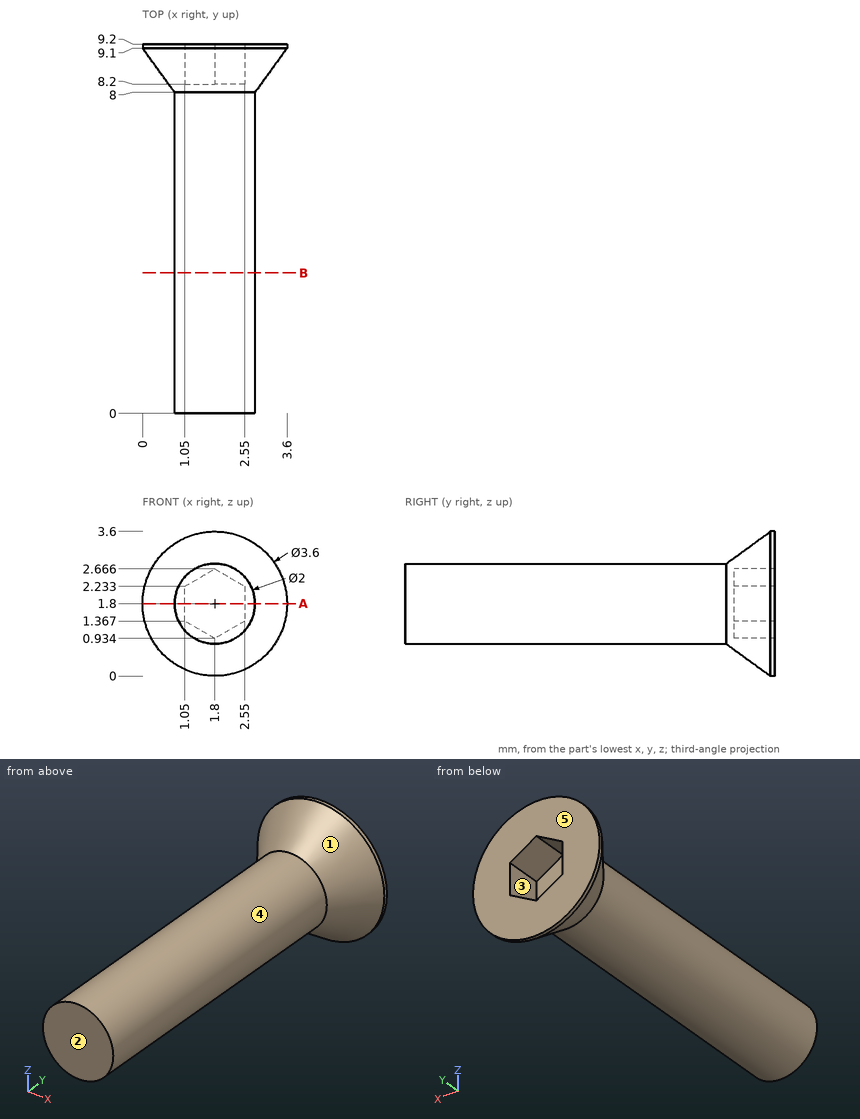
Here's the drawing with two shaded views (mm, measured from the low corner). I have some questions. A direction names the side the tool comes from. Give positions to 0.01 mm unless a question says otherwise; leave off trailing zeros. Loops run counter-clockwise (first coordinate to the right, second up) from the corner with the lowest first, then second, coordinate; pieces in that order, holes last. Notation, with made-up numbers: (0, 57) - (28, 57) arc R14 ccw to (28, 80) - close; hole circle Ø2 at (-27, 47). An arc over 180 degrees is marked (long way). Answer in a Markdown table with one row per item. Add a question column.
Q1. We'd pull the mould along Z, two halves only. Please class the marked faces 1, 2 and 3: +Z half, -Z half, draft (parallel to the pull), parting line (faces both ways), or undercut.
Q2. If we section it at B-B (y = 3.5): List the corners of the cut face in (x, z) for me.
Q3. If we section it at A-A (z = 1.8): List the corners of the cut face in (x, y) for me, plus the area to 3 significant figures.
Q4. Please list where these lines run through material, in increasing order: L1, parallel to Y at x = 1.8, z = 1.85; L2, parallel to X at y = 6, z = 2.3; L3, parallel to Y at x = 2.6, z = 2.6. Write a range as from..to.
Q5. For pin 1 (1 mm diameter, centred on y = 4.5, z = 0.5, fed in from -X); pin 2 (1.5 mm diameter, centred on x = 1, y = 4.5, fed in from +Z); pin 3 (0.5 mm diameter, centred on x = 2, z = 2, fed in from +Y), each with a flat end and sliding along its axis, tell me the tip position at first contact or that it passes through.
Q6. Which directions (+Z, -Z, +X, -X, +Y, -Y) give clear straight access to the entire face, cutting with the end or side of a thin tool? Please do the marked faces 4 and 5.
The answers:
| question | item | result |
|---|---|---|
| 1 | face 1 | parting line |
| 1 | face 2 | draft |
| 1 | face 3 | undercut |
| 2 | outline | circle Ø2 at (1.8, 1.8) |
| 3 | outline | (0, 9.1) - (0.8, 8) - (0.8, 0) - (2.8, 0) - (2.8, 8) - (3.6, 9.1) - (3.6, 9.2) - (2.55, 9.2) - (2.55, 8.2) - (1.05, 8.2) - (1.05, 9.2) - (0, 9.2) - close |
| 3 | area | 17.9 mm^2 |
| 4 | L1 | y = 0..8.2 |
| 4 | L2 | x = 0.93..2.67 |
| 4 | L3 | y = 8.18..9.2 |
| 5 | pin 1 | stops at x = 1.2 |
| 5 | pin 2 | stops at z = 2.8 |
| 5 | pin 3 | stops at y = 8.2 |
| 6 | face 4 | -Y |
| 6 | face 5 | +Z, -Z, +X, -X, +Y |
